CAD build for the part. Positions are in the model's coordinates, mm. Face numbers are marked on the shaded views. A direction names the side the tool comes from. Give positions to 0.01 mm unless a question says otherwise; leave off trailing zeros. Order: outer loops, then holes, each group sorted by start corner. A loop starts at its lowest first (then second) coordinate and runs counter-clockwise, first axis right, second up.
from build123d import *

# Parameters (mm, degrees)
EXTRUDE008_DEPTH = 10
EXTRUDE002_DEPTH = 20


with BuildPart() as extrude008:
    # Sketch006 (on Extrude) → Extrude008 (new body, symmetric)
    with BuildSketch(Plane.XZ):
        with BuildLine():
            ThreePointArc((20.501, -13), (23.751, -9.75), (20.501, -6.5))
            Line((20.501, -6.5), (17.501, -6.5))
            ThreePointArc((17.501, -6.5), (14.251, -9.75), (17.501, -13))
            Line((20.501, -13), (17.501, -13))
        make_face()
    extrude(amount=EXTRUDE008_DEPTH, both=True)


with BuildPart() as shell:
    # Sketch001 (on Sketch) → Extrude002 (new body)
    with BuildSketch(Plane(origin=(0, 0, 0), x_dir=(1, 0, 0), z_dir=(0, 0, -1))):
        with BuildLine():
            Line((3, 65.151), (3, 10.001))
            ThreePointArc((3, 10.001), (5.050485, 5.050192), (10.001, 2.999))
            Line((10.001, 2.999), (103.251, 2.999))
            ThreePointArc((103.251, 2.999), (108.202515, 5.049778), (110.254, 10.001))
            Line((110.251, 65.151), (110.254, 10.001))
            ThreePointArc((110.251, 65.151), (108.200808, 70.101101), (103.251, 72.152))
            Line((10.001, 72.152), (103.251, 72.152))
            ThreePointArc((10.001, 72.152), (5.050545, 70.101455), (3, 65.151))
        make_face()
        with BuildLine():
            Line((5, 65.151), (5.001, 10.001))
            ThreePointArc((5.001, 10.001), (6.465405, 6.465113), (10.001, 5))
            Line((10.001, 5), (103.251, 5.001))
            ThreePointArc((103.251, 5.001), (106.786887, 6.465405), (108.252, 10.001))
            Line((108.252, 10.001), (108.251, 65.151))
            ThreePointArc((108.251, 65.151), (106.786595, 68.686887), (103.251, 70.152))
            Line((103.251, 70.152), (10.001, 70.152))
            ThreePointArc((10.001, 70.152), (6.464759, 68.687241), (5, 65.151))
        make_face(mode=Mode.SUBTRACT)
    extrude(amount=EXTRUDE002_DEPTH)

    # Cut001: cut Extrude008
    add(extrude008.part, mode=Mode.SUBTRACT)


solid = shell.part
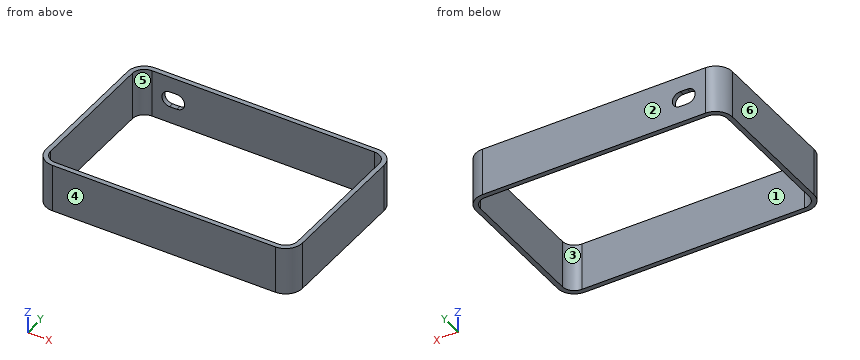
1. 3-axis set-ups, long thin cutter, end or side, ignore diameter. For the marked faces 5 and 6: which of +Z, -Z, +X, -X, +Y, -Y reach the whole face in a straight line?
2. Saw through at D-D on z = -9.75. Give the cut face in (x, y), plus the area to 3 significant figures.
3. Mould opens along Y. For the marked faces 1, 2, 3 and 4 say: released by +Y, released by -Y, zero draft, split by the parting line, or undercut.
4. Wall check: line 1 (Y direction, x = 99.5, z = -15.5); line 2 (X direction, y = -13, z = -11); line 3 (Y direction, x = 103.5, z = -7.25). Give the ranges that are in metal, low to high.
5. Pin check, flat tip, straight feed: P1, Ø1, axis at x = 18.5, y = -4, coming from the +Z side. Stop position of the tip, or through.
6. Saw through at A-A on z = -4. Give the cut face in (x, y), plus the area to 3 significant figures.
7. Saw through at C-C on x = 76. Give the cut face in (y, z).
8. Saw through at B-B on y = -19. Give the cut face in (x, z), plus the area to 4 significant figures.
Reported:
1. face 5: +Z, -Z
1. face 6: +Z, -Z, -X, +Y, -Y
2. outline: (3, -65.15) arc R7 ccw to (10, -72.15) - (103.25, -72.15) arc R7 ccw to (110.25, -65.15) - (110.25, -10) arc R7 ccw to (103.25, -3) - (23.75, -3) - (23.75, -5) - (103.25, -5) arc R5 cw to (108.25, -10) - (108.25, -65.15) arc R5 cw to (103.25, -70.15) - (10, -70.15) arc R5 cw to (5, -65.15) - (5, -10) arc R5 cw to (10, -5) - (14.25, -5) - (14.25, -3) - (10, -3) arc R7 ccw to (3, -10) - close
2. area: 650 mm2
3. face 1: undercut
3. face 2: released by +Y
3. face 3: undercut
3. face 4: released by -Y
4. line 1: y = -72.15 to -70.15, -5 to -3
4. line 2: x = 3 to 5, 108.25 to 110.25
4. line 3: y = -72.15 to -70.15, -5.01 to -3
5. P1: stops at z = 0
6. outline: (3, -65.15) arc R7 ccw to (10, -72.15) - (103.25, -72.15) arc R7 ccw to (110.25, -65.15) - (110.25, -10) arc R7 ccw to (103.25, -3) - (10, -3) arc R7 ccw to (3, -10) - close; hole (5, -65.15) arc R5 ccw to (10, -70.15) - (103.25, -70.15) arc R5 ccw to (108.25, -65.15) - (108.25, -10) arc R5 ccw to (103.25, -5) - (10, -5) arc R5 ccw to (5, -10) - close
6. area: 669 mm2
7. outline: (-72.15, -20) - (-70.15, -20) - (-70.15, 0) - (-72.15, 0) - close; (-5, -20) - (-3, -20) - (-3, 0) - (-5, 0) - close
8. outline: (3, -20) - (5, -20) - (5, 0) - (3, 0) - close; (108.25, -20) - (110.25, -20) - (110.25, 0) - (108.25, 0) - close
8. area: 80.05 mm2
